from build123d import *

# Parameters (mm, degrees)
SKETCH1_R               = 1.09
BOSS_EXTRUDE1_DEPTH     = 32.2
BOSS_EXTRUDE2_DEPTH     = 14
CUT_EXTRUDE1_DEPTH      = 45.341177251
CUT_EXTRUDE1_DEPTH_BACK = 45.341177251
SKETCH3_W               = 7
SKETCH3_H               = 2.6


with BuildPart() as part:
    # Sketch1 → Boss-Extrude1 (new body)
    with BuildSketch(Plane(origin=(0, 0, 0), x_dir=(0, 0, -1), z_dir=(1, 0, 0))):
        Circle(SKETCH1_R)
    extrude(amount=BOSS_EXTRUDE1_DEPTH)

    # Sketch2 → Boss-Extrude2 (add)
    with BuildSketch(Plane(origin=(30.2, 0, 0), x_dir=(0, 0, -1), z_dir=(1, 0, 0))):
        with BuildLine():
            Line((-1.5, -2.5), (1.5, -2.5))
            ThreePointArc((1.5, -2.5), (2.207106781, -2.207106781), (2.5, -1.5))
            Line((2.5, -1.5), (2.5, 1.5))
            ThreePointArc((2.5, 1.5), (2.207106781, 2.207106781), (1.5, 2.5))
            Line((1.5, 2.5), (-1.5, 2.5))
            ThreePointArc((-1.5, 2.5), (-2.207106781, 2.207106781), (-2.5, 1.5))
            Line((-2.5, 1.5), (-2.5, -1.5))
            ThreePointArc((-2.5, -1.5), (-2.207106781, -2.207106781), (-1.5, -2.5))
        make_face()
    extrude(amount=BOSS_EXTRUDE2_DEPTH)

    # Sketch3 → Cut-Extrude1 (cut, two sides: drawn at the far end of the back side and taken through both)
    with BuildSketch(Plane(origin=(0, 0, 0), x_dir=(1, 0, 0), z_dir=(0, 1, 0)).offset(-CUT_EXTRUDE1_DEPTH_BACK)):
        with Locations((41.7, 0)):
            Rectangle(SKETCH3_W, SKETCH3_H)
    extrude(amount=CUT_EXTRUDE1_DEPTH + CUT_EXTRUDE1_DEPTH_BACK, mode=Mode.SUBTRACT)


solid = part.part
Read the model definition and answer for the solid it produces. Units are mm, in the model's axes. A direction names the side the tool comes from. Give positions to 0.01 mm unless a question says otherwise; leave off trailing zeros. Loops run counter-clockwise (first coordinate to the right, second up) from the corner with the lowest first, then second, coordinate; pieces in that order, holes last. Notation, with made-up numbers: M 38,42.25 L 50,42.25 A17 ccw 50,71.25 Z; hole C -33.75,-39.75 d4. An arc over 180 degrees is marked long. Write each question's results on one line, items separated by ' | '.
1. A tool of negligible diameter and unlimited length cuts with its end or side. For faces 4 (the face through (14.889, -1.064, 0.236)), 5 (the face through (41, 0, -1.3)), 6 (the face through (36, -2.5, 0)), from which of +Z, -Z, +X, -X, +Y, -Y can it reach the whole face along a straight path? Write none if from no direction.
Values:
face 4: -X | face 5: +X, +Y, -Y | face 6: +Z, -Z, +X, -X, -Y
2. The mould has two halves that part along Z. Classify faces 1 (the face through (38.2, 0, 0)), 2 (the face through (44.2, 0, -2)), 3 (the face through (37.102, -2.215, -2.199)): pulls with the +Z half, pulls with the -Z half, needs draft (parallel to the pull), parting line crosses it, or undercut.
Values:
face 1: undercut | face 2: needs draft | face 3: pulls with the -Z half
3. Section B-B on z = 0 is taken. Give the vertices of the cut face in (x, y), plus the area to 3 significant figures.
Values:
outline: M 0,-1.09 L 30.2,-1.09 L 30.2,-2.5 L 38.2,-2.5 L 38.2,2.5 L 30.2,2.5 L 30.2,1.09 L 0,1.09 Z | area: 106 mm^2
4. Section C-C on y = 0 is taken. Give the vertices of the cut face in (x, z).
Values:
outline: M 0,-1.09 L 30.2,-1.09 L 30.2,-2.5 L 44.2,-2.5 L 44.2,-1.3 L 38.2,-1.3 L 38.2,1.3 L 44.2,1.3 L 44.2,2.5 L 30.2,2.5 L 30.2,1.09 L 0,1.09 Z
5. Section D-D on x = 15 is taken. Give the vertices of the cut face in (y, z), plus the area to 3 significant figures.
Values:
outline: C 0,0 d2.18 | area: 3.73 mm^2
6. Straight lines are drawn through the part: line 1 (Z direction, x = 42.5, y = -1.4); line 2 (X direction, y = 1.5, z = -0.95); line 3 (Y direction, x = 19.5, z = 0.1). For each, find the intervals that lie inside material, in ascending order. Write a range as [from, to].
Values:
line 1: z = [-2.5, -1.3], [1.3, 2.5] | line 2: x = [30.2, 38.2] | line 3: y = [-1.09, 1.09]
7. Section A-A on x = 40 is taken. Give the vertices of the cut face in (y, z).
Values:
outline: M -2.5,-1.5 A1 ccw -1.5,-2.5 L 1.5,-2.5 A1 ccw 2.5,-1.5 L 2.5,-1.3 L -2.5,-1.3 Z; M -2.5,1.3 L 2.5,1.3 L 2.5,1.5 A1 ccw 1.5,2.5 L -1.5,2.5 A1 ccw -2.5,1.5 Z
8. Given pin 1 (1.3 mm diameter, centred on y = -0.5, z = -0.5, fed in from +X); pin 2 (3 mm diameter, centred on x = 21.5, y = 0.5, fed in from +Z); pin 3 (1.5 mm diameter, centred on x = 19.5, z = 1, fed in from +Y), each flat-ended and moving along its own axis, determine where each tip first touches the part or whether it passes through.
Values:
pin 1: stops at x = 38.2 | pin 2: stops at z = 1.09 | pin 3: stops at y = 1.06
